Model file for the job. Use its own axes, mm. A direction names the side the tool comes from. Give positions to 0.01 mm unless a question says otherwise; leave off trailing zeros. Order: outer loops, then holes, each group sorted by start corner. A loop starts at its lowest first (then second) coordinate and runs counter-clockwise, first axis right, second up. Notation, with made-up numbers: (-32, -1.5) -> (12, -1.5) arc R32 cw to (12, 27.5) -> close; hole circle Ø1 at (87, -30). An arc over 180 degrees is marked (long way). Answer in a Markdown table with one row per item. Add a question column.
from build123d import *

# Parameters (mm, degrees)
F1_DEPTH = 30
F3_R     = 3
F4_DEPTH = 25
F5_DEPTH = 5
F6_W     = 15
F6_H     = 14
F7_DEPTH = 160
F8_R     = 5
F2_W     = 30
F2_H     = 12
F2_R     = 1.35
F9_DEPTH = 25


# Not quite as in the source:
# - a feature names something its author has since deleted; it is built from what else it names


with BuildPart() as f1:
    # F0 (on Top) → F1 (new body)
    with BuildSketch(Plane.XY):
        Polygon((29, 5), (8, 32), (-8, 32), (-29, 5), (-69, 5), (-69, 0), (-26, 0), (-8, 22), (8, 22), (26, 0), (69, 0), (69, 5), align=None)
    extrude(amount=F1_DEPTH)

    # F3 (on face) → F4 (cut)
    with BuildSketch(Plane.XZ.offset(-22)):
        with Locations((0, 15)):
            Circle(F3_R)
    extrude(amount=-F4_DEPTH, mode=Mode.SUBTRACT)

    # F3 (on face) → F5 (cut)
    with BuildSketch(Plane.XZ.offset(-22)):
        Polygon((0, 9.1687622812), (5.05, 12.0843811406), (5.05, 17.9156188594), (0, 20.8312377188), (-5.05, 17.9156188594), (-5.05, 12.0843811406), align=None)
        with Locations((0, 15)):
            Circle(F3_R, mode=Mode.SUBTRACT)
    extrude(amount=-F5_DEPTH, mode=Mode.SUBTRACT)

    # F6 (on face) → F7 (cut)
    with BuildSketch(Plane.YZ.offset(69)):
        with Locations((12.5, 15)):
            Rectangle(F6_W, F6_H)
    extrude(amount=-F7_DEPTH, mode=Mode.SUBTRACT)

    # F8
    f8_edges = [f1.edges().sort_by_distance(p)[0] for p in [
        (-8, 32, 15),
        (8, 32, 15),
        (-8, 22, 15),
        (8, 22, 15),
        (29, 5, 26),
        (29, 5, 4),
        (13.484848, 20, 8),
        (13.484848, 20, 22),
        (-13.484848, 20, 8),
        (-13.484848, 20, 22),
        (-29, 5, 4),
        (-29, 5, 26),
        (-69, 2.5, 30),
        (-69, 2.5, 0),
        (69, 2.5, 30),
        (69, 2.5, 0),
    ]]
    fillet(f8_edges, radius=F8_R)

    # F2 (on face) → F9 (cut)
    with BuildSketch(Plane(origin=(0, 5, 0), x_dir=(-1, 0, 0), z_dir=(0, 1, 0))):
        with Locations((47, 15)):
            Rectangle(F2_W, F2_H)
        with Locations((-47, 15)):
            Rectangle(F2_W, F2_H)
        with BuildLine():
            Line((-29, 13.65), (-29, 16.35))
            ThreePointArc((-29, 16.35), (-30.35, 15), (-29, 13.65))
        make_face()
        with BuildLine():
            ThreePointArc((-29, 13.65), (-28.0454058454, 14.0454058454), (-27.65, 15))
            ThreePointArc((-27.65, 15), (-28.0454058454, 15.9545941546), (-29, 16.35))
            Line((-29, 16.35), (-29, 13.65))
        make_face()
        with Locations((-65, 15)):
            Circle(F2_R)
        with Locations((29, 15)):
            Circle(F2_R)
        with Locations((65, 15)):
            Circle(F2_R)
    extrude(amount=-F9_DEPTH, mode=Mode.SUBTRACT)


solid = f1.part
Item 1: Saw through at A-A on x = 50.5. List the corners of the cut face in (y, z), plus the area to 3 significant figures.
Item 2: Saw through at B-B on z = 6.75. List the corners of the cut face in (x, y).
Item 3: Pin check, flat tips, straight feed: pin 1 Ø1.5 at (y, z) = (7.5, 21) entering from +X (3 decimals); pin 2 Ø3 at (y, z) = (28, 11) entering from +X; pin 3 Ø3.5 at (x, z) = (-65, 15) entering from +Y; pin 4 Ø12 at (y, z) = (22, 16.5) entering from -X. Stop position of each tip, or through.
Item 4: Two-plate mould, pull along Z, no slides. Class faces 6 (the cylindrical face through (63.712, 2.535, 15.406)), 7 (the cylindrical face through (-68, 2, 2)), 8 (the cylindrical face through (-29.277, 5.495, 26.056)): pulls with the +Z half, pulls with the -Z half, needs draft (parallel to the pull), parting line crosses it, or undercut.
Item 5: Saw through at C-C on y = 13.5. List the corners of the cut face in (x, z).
Item 6: Which spindle directions (+Z, -Z, +X, -X, +Y, -Y) get a long thin tool onto all of the face, cutting with end or side? Do faces 1 (the cylindrical face through (15, 19, 20)), 2 (the cylindrical face through (-7.744, 21.532, 15.21)), 3 (the flat face through (-62, 3, 15)), 4 (the flat face through (69, 2, 15)), 5 (the flat face through (5.05, 24, 15)). Say none if no direction does.
Item 7: Wall check: line 1 (Z direction, x = 32.5, y = 4.5); line 2 (Y direction, x = -5.5, z = 19.5); line 3 (Y direction, x = 56, z = 4.5). Give the ranges that are in metal, low to high.
Item 8: Saw through at D-D on x = 24. List the corners of the cut face in (y, z).
Evaluation:
| question | item | result |
|---|---|---|
| 1 | outline | (0, 0) -> (5, 0) -> (5, 9) -> (0, 9) -> close; (0, 21) -> (5, 21) -> (5, 30) -> (0, 30) -> close |
| 1 | area | 90.0 mm2 |
| 2 | outline | (-69, 0) -> (-26, 0) -> (-9.5, 20.17) arc R5 cw to (-5.63, 22) -> (5.63, 22) arc R5 cw to (9.5, 20.17) -> (26, 0) -> (69, 0) -> (69, 5) -> (31.45, 5) arc R5 cw to (27.5, 6.93) -> (9.5, 30.07) arc R5 ccw to (5.55, 32) -> (-5.55, 32) arc R5 ccw to (-9.5, 30.07) -> (-27.5, 6.93) arc R5 cw to (-31.45, 5) -> (-69, 5) -> close |
| 3 | pin 1 | passes through |
| 3 | pin 2 | stops at x = 12.28 |
| 3 | pin 3 | stops at y = 5 |
| 3 | pin 4 | stops at x = -18.88 |
| 4 | face 6 | undercut |
| 4 | face 7 | pulls with the -Z half |
| 4 | face 8 | needs draft |
| 5 | outline | (-22.39, 0) -> (-14.95, 0) -> (-14.95, 8) -> (-22.39, 8) -> close; (-22.39, 22) -> (-14.95, 22) -> (-14.95, 30) -> (-22.39, 30) -> close; (14.95, 0) -> (22.39, 0) -> (22.39, 8) -> (14.95, 8) -> close; (14.95, 22) -> (22.39, 22) -> (22.39, 30) -> (14.95, 30) -> close |
| 6 | face 1 | +X, -X, -Y |
| 6 | face 2 | +Z, -Z, -Y |
| 6 | face 3 | +Y, -Y |
| 6 | face 4 | +Z, -Z, +X, +Y, -Y |
| 6 | face 5 | -Y |
| 7 | line 1 | z = 0 to 9, 21 to 30 |
| 7 | line 2 | y = 22 to 32 |
| 7 | line 3 | y = 0 to 5 |
| 8 | outline | (2.44, 0) -> (11.43, 0) -> (11.43, 8) -> (5, 8) -> (5, 22) -> (11.43, 22) -> (11.43, 30) -> (2.44, 30) -> close |
